For this review, take the finished solid that the model builds, in its own axes (mm). Give positions to 0.01 mm unless a question says otherwise; leave off trailing zeros. Order: outer loops, then holes, each group sorted by start corner. A loop starts at its lowest first (then second) coordinate and runs counter-clockwise, first axis right, second up. Notation, with made-up numbers: M -10,-0.5 L 22,-0.5 A24 cw 22,19.5 Z; hole C -9,-0.75 d11. An arc over 180 degrees is marked long. Answer as CSV lines item,"result". Start each with the question number.
1. We need section D-D, the plane y = 1.55. State how many separate pieces and enclosed holes the cut face has, and give its area (3 significant figures).
2. We need section A-A, the plane z = -14. Give the boundary of the cut face in (x, y).
3. We need section C-C, the plane x = 23.57. Give the boundary of the cut face in (y, z).
4. Clearance check with flat-ended pins moving along their axes: P1, Ø1.6, axis at x = -32, y = 2.5, coming from the +Z side; P2, Ø1.2, axis at x = -40, y = 1.5, coming from the +Z side; P3, Ø1, axis at x = 21.5, y = 1, coming from the -Z side. State where each tip first meets the part, or that it passes through.
5. We need section B-B, the plane x = -27. Give the boundary of the cut face in (y, z), and give its area (3 significant figures).
6. For line 1 along X through (y, z) = (1.4, 0); line 2 along X through (y, z) = (1.6, 31.5); line 3 along Z through (x, y) = (1, 1.2), list the stretches that pass through material, from the lowest coordinate up.
from build123d import *

# Parameters (mm, degrees)
SKETCH_1_R          = 52
SKETCH_1_R_2        = 29
SKETCH_1_R_3        = 2.05
SKETCH_1_R_4        = 2.1
EXTRUDE_1_DEPTH     = 4
SKETCH_2_W          = 182
SKETCH_2_H          = 210.035227354
SKETCH_2_W_2        = 82
SKETCH_2_H_2        = 110.035227354
CUT_EXTRUDE_1_DEPTH = 4


with BuildPart() as part:
    # 草图1 → 凸台-拉伸1 (new body)
    with BuildSketch(Plane(origin=(0, 0, 0), x_dir=(1, 0, 0), z_dir=(0, 1, 0))):
        with Locations(Location((0, 0, 0), (0, 0, 270))):
            Circle(SKETCH_1_R)
        with Locations(Location((0, 0, 0), (0, 0, 270))):
            Circle(SKETCH_1_R_2, mode=Mode.SUBTRACT)
        with Locations(Location((47, 0, 0), (0, 0, 270))):
            Circle(SKETCH_1_R_3, mode=Mode.SUBTRACT)
        with Locations(Location((33.234018716, -33.234018716, 0), (0, 0, 270))):
            Circle(SKETCH_1_R_3, mode=Mode.SUBTRACT)
        with Locations(Location((0, -47, 0), (0, 0, 270))):
            Circle(SKETCH_1_R_3, mode=Mode.SUBTRACT)
        with Locations(Location((-33.234018716, -33.234018716, 0), (0, 0, 270))):
            Circle(SKETCH_1_R_3, mode=Mode.SUBTRACT)
        with Locations(Location((-47, 0, 0), (0, 0, 270))):
            Circle(SKETCH_1_R_3, mode=Mode.SUBTRACT)
        with Locations(Location((-33.234018716, 33.234018716, 0), (0, 0, 270))):
            Circle(SKETCH_1_R_3, mode=Mode.SUBTRACT)
        with Locations(Location((0, 47, 0), (0, 0, 270))):
            Circle(SKETCH_1_R_3, mode=Mode.SUBTRACT)
        with Locations(Location((33.234018716, 33.234018716, 0), (0, 0, 270))):
            Circle(SKETCH_1_R_3, mode=Mode.SUBTRACT)
        with Locations(Location((-23.57, 23.57, 0), (0, 0, 270))):
            Circle(SKETCH_1_R_4, mode=Mode.SUBTRACT)
        with Locations(Location((-23.57, -23.57, 0), (0, 0, 270))):
            Circle(SKETCH_1_R_4, mode=Mode.SUBTRACT)
        with Locations(Location((23.57, -23.57, 0), (0, 0, 90))):
            Circle(SKETCH_1_R_4, mode=Mode.SUBTRACT)
        with Locations(Location((23.57, 23.57, 0), (0, 0, 90))):
            Circle(SKETCH_1_R_4, mode=Mode.SUBTRACT)
        Polygon((37, -9.55), (37, -11), (33.8, -11), (33.8, -9.55), (33.8, -5.45), (33.8, -4), (37, -4), (37, -5.45), (41, -5.45), (41, -9.55), align=None, mode=Mode.SUBTRACT)
        Polygon((37, 20.45), (37, 19), (33.8, 19), (33.8, 20.45), (30.6, 20.45), (30.6, 24.55), (33.8, 24.55), (33.8, 26), (37, 26), (37, 24.55), (41, 24.55), (41, 20.45), align=None, mode=Mode.SUBTRACT)
        Polygon((-33.8, 26), (-37, 26), (-37, 24.55), (-41, 24.55), (-41, 20.45), (-37, 20.45), (-37, 19), (-33.8, 19), (-33.8, 20.45), (-30.6, 20.45), (-30.6, 24.55), (-33.8, 24.55), align=None, mode=Mode.SUBTRACT)
        Polygon((-33.8, -4), (-37, -4), (-37, -5.45), (-41, -5.45), (-41, -9.55), (-37, -9.55), (-37, -11), (-33.8, -11), (-33.8, -9.55), (-33.8, -5.45), align=None, mode=Mode.SUBTRACT)
    extrude(amount=EXTRUDE_1_DEPTH)

    # 草图2 → 切除-拉伸-薄壁1 (cut)
    with BuildSketch(Plane(origin=(0, 4, 0), x_dir=(1, 0, 0), z_dir=(0, 1, 0))):
        Rectangle(SKETCH_2_W, SKETCH_2_H)
        Rectangle(SKETCH_2_W_2, SKETCH_2_H_2, mode=Mode.SUBTRACT)
    extrude(amount=-CUT_EXTRUDE_1_DEPTH, mode=Mode.SUBTRACT)


solid = part.part
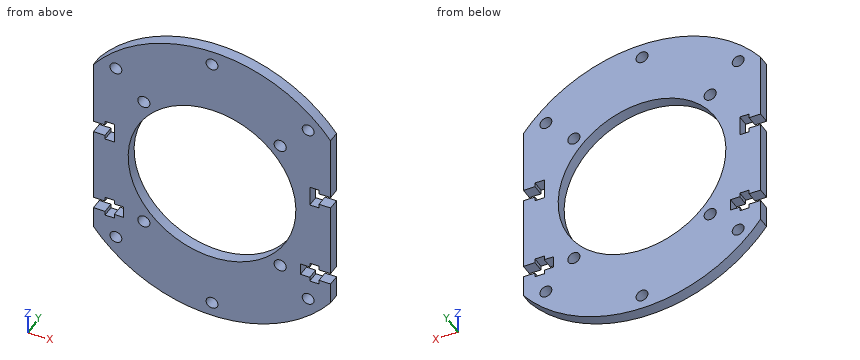
Result set:
1,separate pieces,"1"
1,enclosed holes,"11"
1,area,"4,580 mm2"
2,outline,"M -41,0 L -25.4,0 L -25.4,4 L -41,4 Z; M 25.4,0 L 41,0 L 41,4 L 25.4,4 Z"
3,outline,"M 0,-46.35 L 4,-46.35 L 4,-25.67 L 0,-25.67 Z; M 0,-21.47 L 4,-21.47 L 4,-16.9 L 0,-16.9 Z; M 0,16.9 L 4,16.9 L 4,21.47 L 0,21.47 Z; M 0,25.67 L 4,25.67 L 4,46.35 L 0,46.35 Z"
4,P1,"z = 41.6"
4,P2,"z = 33.94"
4,P3,"z = -47.57"
5,outline,"M 0,-44.44 L 4,-44.44 L 4,-10.58 L 0,-10.58 Z; M 0,10.58 L 4,10.58 L 4,44.44 L 0,44.44 Z"
5,area,"271 mm2"
6,line 1,"-41 to -29, 29 to 41"
6,line 2,"-41 to -34.33, -32.14 to 32.14, 34.33 to 41"
6,line 3,"-51.99 to -48.79, -45.21 to -28.98, 28.98 to 45.21, 48.79 to 51.99"
